```python
from build123d import *

# Parameters (mm, degrees)
F0_R     = 2.5
F0_R_2   = 0.25
F1_DEPTH = 4.5
F0_R_3   = 2.875
F2_DEPTH = 1
F3_DEPTH = 10


with BuildPart() as f1:
    # F0 (on Top) → F1 (new body)
    with BuildSketch(Plane.XY):
        Circle(F0_R)
        with Locations((-1.25, 0)):
            Circle(F0_R_2, mode=Mode.SUBTRACT)
        with Locations((1.25, 0)):
            Circle(F0_R_2, mode=Mode.SUBTRACT)
        with Locations((-1.25, 0)):
            Circle(F0_R_2)
        with Locations((1.25, 0)):
            Circle(F0_R_2)
    extrude(amount=F1_DEPTH)

    # F0 (on Top) → F2 (join)
    with BuildSketch(Plane.XY):
        Circle(F0_R_3)
        Circle(F0_R, mode=Mode.SUBTRACT)
    extrude(amount=F2_DEPTH)

    # F0 (on Top) → F3 (join)
    with BuildSketch(Plane.XY):
        with Locations((-1.25, 0)):
            Circle(F0_R_2)
        with Locations((1.25, 0)):
            Circle(F0_R_2)
    extrude(amount=-F3_DEPTH)


solid = f1.part
```
CAD build for the part. Positions are in the model's coordinates, mm. A direction names the side the tool comes from. Coordinates: 2 decimals unless noted, no trailing zeros. Write each loop counter-clockwise with the first axis right and the second up, starting at its lowest first coordinate (ties: lowest second). Pieces come first, ordered by that corner, then holes.
(1) Drill centre lines: probe 1 along Z at (x, y) = (0.3, -1.2); probe 2 along Z at (x, y) = (-0.5, -2.6); probe 3 along Y at (x, z) = (1.15, -0.5). Where is each one in solid material? Low to high.
(2) Cut at B-B, the plane y = 0. List the corners of the cut face in (x, z) (3 decimals), and give its area (4 significant figures).
(3) Cut at A-A, the plane x = 0. List the corners of the cut face in (y, z) (3 decimals), and give its area (4 significant figures).
(4) Cut at D-D, the plane y = -2.15. List the corners of the cut face in (x, z), and give its area (3 significant figures).
(5) 3-axis set-ups, long thin cutter, end or side, ignore diameter. For faces 1 (the face through (-0.37, 2.85, 0.49)), 2 (the face through (-0.54, -2.44, 2.73)): which of +Z, -Z, +X, -X, +Y, -Y reach the whole face in a straight line?
(6) Flat gauge pins, fed straight in: pin 1 (3 mm diameter, centred on x = -0.5, z = -5, fed in from +Y); pin 2 (3 mm diameter, centred on y = -0.5, z = -7, fed in from -X). Where does each tip first touch, or does it go through?
(7) Cut at C-C, the plane z = 0.5. List the corners of the cut face in (x, y) (3 decimals), and give its area (3 significant figures).
Geometry says:
1. probe 1: z = 0 to 4.5
1. probe 2: z = 0 to 1
1. probe 3: y = -0.23 to 0.23
2. outline: (-2.875, 0) - (-1.5, 0) - (-1.5, -10) - (-1, -10) - (-1, 0) - (1, 0) - (1, -10) - (1.5, -10) - (1.5, 0) - (2.875, 0) - (2.875, 1) - (2.5, 1) - (2.5, 4.5) - (-2.5, 4.5) - (-2.5, 1) - (-2.875, 1) - close
2. area: 33.25 mm2
3. outline: (-2.875, 0) - (2.875, 0) - (2.875, 1) - (2.5, 1) - (2.5, 4.5) - (-2.5, 4.5) - (-2.5, 1) - (-2.875, 1) - close
3. area: 23.25 mm2
4. outline: (-1.91, 0) - (1.91, 0) - (1.91, 1) - (1.28, 1) - (1.28, 4.5) - (-1.28, 4.5) - (-1.28, 1) - (-1.91, 1) - close
4. area: 12.7 mm2
5. face 1: +Z, -Z
5. face 2: +Z
6. pin 1: stops at y = 0.25
6. pin 2: stops at x = -1.5
7. outline: circle Ø5.75 at (0, 0)
7. area: 26.0 mm2
